Could you check a few things on this model? Use its own coordinates, in mm. Face numbers are marked on the shaded views. A direction names the side the tool comes from. Round coordinates to 2 decimals unless told otherwise and drop trailing zeros. Loops run counter-clockwise (first coordinate to the right, second up) from the corner with the lowest first, then second, coordinate; pieces in that order, holes last. Notation, with made-up numbers: (70.5, 64.5) - (96.5, 64.5) arc R22 cw to (96.5, 103.5) - close; hole circle Ø4 at (30.5, -29). An arc over 180 degrees is marked (long way). Answer as CSV lines item,"result". Start each with the question number.
1) We'd pull the mould along X, two halves only. Please class the marked faces 1, 2, 3 and 4: pulls with the +X half, pulls with the -X half, needs draft (parallel to the pull), parting line crosses it, or undercut.
2) Suppose I cut it at A-A, the plane z = 1.5. Count the separate pieces of the cut face and the enclosed holes in it, then the cut area to 3 significant figures.
3) Suppose I cut it at C-C, the plane y = 18. Write out the boundary of the cut face in (x, z), then the cut area to 3 significant figures.
4) Suppose I cut it at B-B, the plane x = 0. Write out the boundary of the cut face in (y, z).
5) Suppose I cut it at D-D, the plane x = 18. Write out the boundary of the cut face in (y, z).
6) I'm going to push flat-ended pins straight in: pin 1 Ø5 at (x, y) = (15.59, -9) entering from -Z; pin 2 Ø1 at (x, z) = (-19.5, 5) entering from +Y; pin 3 Ø6 at (x, z) = (8, 7) entering from +Y; pin 4 Ø1.5 at (y, z) = (18, 4) entering from -X. Where does each tip first touch, or does it pass through?
7) Please list where these lines run through material, in increasing order: line 1 along Y through (x, z) = (-10, 0.95); line 2 along Y through (x, z) = (1, 2); line 3 along Z through (x, y) = (4.5, 8).
8) Which directions (+Z, -Z, +X, -X, +Y, -Y) give clear straight access to the entire face, cutting with the end or side of a thin tool? Please do the marked faces 5 and 6.
```python
from build123d import *

# Parameters (mm, degrees)
SKETCH_R        = 31.5
SKETCH_R_2      = 4
PAD_DEPTH       = 3
SKETCH001_R     = 21
SKETCH001_R_2   = 14.5
PAD001_DEPTH    = 10
SKETCH002_R     = 14.5
SKETCH002_R_2   = 4
PAD002_DEPTH    = 2
SKETCH003_R     = 6.5
SKETCH003_R_2   = 4
PAD003_DEPTH    = 8
SKETCH005_R     = 2.5
SKETCH005_R_2   = 1.5
POCKET001_DEPTH = 3.001
SKETCH008_R     = 1.5
POCKET_DEPTH    = 13.001
SKETCH007_R     = 1.5
POCKET002_DEPTH = 13.001
CHAMFER_SIZE    = 1.5
CHAMFER001_SIZE = 1


with BuildPart() as part:
    # Sketch → Pad (new body)
    with BuildSketch(Plane.XY):
        Circle(SKETCH_R)
        Circle(SKETCH_R_2, mode=Mode.SUBTRACT)
    extrude(amount=PAD_DEPTH)

    # Sketch001 (on Face4 of Pad) → Pad001 (join)
    with BuildSketch(Plane.XY.offset(3)):
        Circle(SKETCH001_R)
        Circle(SKETCH001_R_2, mode=Mode.SUBTRACT)
    extrude(amount=PAD001_DEPTH)

    # Sketch002 (on Face6 of Pad001) → Pad002 (join)
    with BuildSketch(Plane.XY.offset(3)):
        Circle(SKETCH002_R)
        Circle(SKETCH002_R_2, mode=Mode.SUBTRACT)
    extrude(amount=PAD002_DEPTH)

    # Sketch003 (on Face8 of Pad002) → Pad003 (join)
    with BuildSketch(Plane.XY.offset(5)):
        Circle(SKETCH003_R)
        Circle(SKETCH003_R_2, mode=Mode.SUBTRACT)
    extrude(amount=PAD003_DEPTH)

    # Sketch005 (on Face3 of Pad001) → Pocket001 (cut, through all)
    with BuildSketch(Plane.XY.offset(3)):
        with Locations((-10, 25)):
            Circle(SKETCH005_R)
        with Locations((10, -25)):
            Circle(SKETCH005_R)
        with Locations((-10, -15)):
            Circle(SKETCH005_R_2)
        with Locations((10, 15)):
            Circle(SKETCH005_R_2)
    extrude(amount=-POCKET001_DEPTH, mode=Mode.SUBTRACT)

    # Sketch008 → Pocket (cut, through all)
    with BuildSketch(Plane.XY.offset(13)):
        with Locations((0, 18)):
            Circle(SKETCH008_R)
        with Locations((-15.588457, -9)):
            Circle(SKETCH008_R)
        with Locations((15.588457, -9)):
            Circle(SKETCH008_R)
    extrude(amount=-POCKET_DEPTH, mode=Mode.SUBTRACT)

    # Sketch007 (on Face13 of Pocket001) → Pocket002 (cut, through all)
    with BuildSketch(Plane.XY.offset(13)):
        with Locations((10, 15)):
            Circle(SKETCH007_R)
        with Locations((-10, -15)):
            Circle(SKETCH007_R)
    extrude(amount=-POCKET002_DEPTH, mode=Mode.SUBTRACT)

    # Chamfer
    chamfer_edges = [part.edges().sort_by_distance(p)[0] for p in [
        (-14.5, 0, 13),
    ]]
    chamfer(chamfer_edges, length=CHAMFER_SIZE)

    # Chamfer001
    chamfer001_edges = [part.edges().sort_by_distance(p)[0] for p in [
        (-6.5, 0, 13),
    ]]
    chamfer(chamfer001_edges, length=CHAMFER001_SIZE)


solid = part.part
```
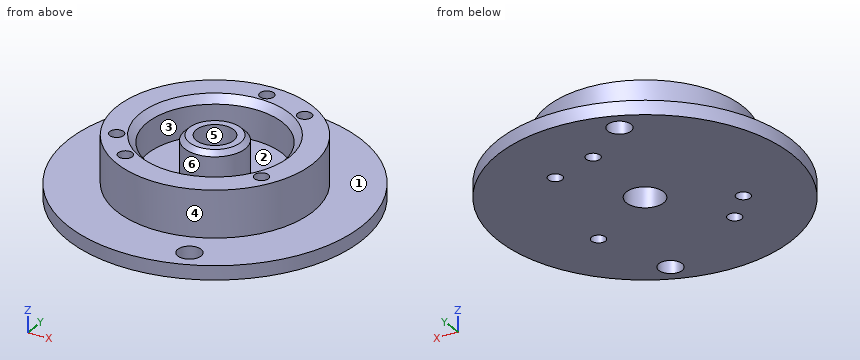
Filled sheet:
1,face 1,"needs draft"
1,face 2,"undercut"
1,face 3,"undercut"
1,face 4,"parting line crosses it"
2,separate pieces,"1"
2,enclosed holes,"8"
2,area,"2,990 mm²"
3,outline,"(-25.85, 0) - (-1.5, 0) - (-1.5, 13) - (-10.82, 13) - (-10.82, 3) - (-25.85, 3) - close; (1.5, 0) - (25.85, 0) - (25.85, 3) - (10.82, 3) - (10.82, 13) - (1.5, 13) - close"
3,area,"332 mm²"
4,outline,"(-31.5, 0) - (-4, 0) - (-4, 13) - (-5.5, 13) - (-6.5, 12) - (-6.5, 5) - (-14.5, 5) - (-14.5, 11.5) - (-16, 13) - (-21, 13) - (-21, 3) - (-31.5, 3) - close; (4, 0) - (16.5, 0) - (16.5, 13) - (16, 13) - (14.5, 11.5) - (14.5, 5) - (6.5, 5) - (6.5, 12) - (5.5, 13) - (4, 13) - close; (19.5, 0) - (31.5, 0) - (31.5, 3) - (21, 3) - (21, 13) - (19.5, 13) - close"
5,outline,"(-25.85, 0) - (25.85, 0) - (25.85, 3) - (10.82, 3) - (10.82, 13) - (-10.82, 13) - (-10.82, 3) - (-25.85, 3) - close"
6,pin 1,"z = 0"
6,pin 2,"y = 8.94"
6,pin 3,"y = 20.4"
6,pin 4,"x = -11.98"
7,line 1,"-29.87 to -16.5, -13.5 to 22.5, 27.5 to 29.87"
7,line 2,"-31.48 to -3.87, 3.87 to 16.88, 19.12 to 31.48"
7,line 3,"0 to 5"
8,face 5,"+Z, -Z"
8,face 6,"+Z"
